from build123d import *

# Parameters (mm, degrees)
BOSS_EXTRUDE1_DEPTH     = 8
CUT_EXTRUDE1_START      = 8
CUT_EXTRUDE1_DEPTH      = 3
SKETCH1_12_R            = 1.7
CUT_EXTRUDE2_DEPTH      = 4
CUT_EXTRUDE3_DEPTH      = 230.948791245
CUT_EXTRUDE3_DEPTH_BACK = 230.948791245
SKETCH1_13_R            = 1.7


with BuildPart() as part:
    # Sketch1 → Boss-Extrude1 (new body)
    with BuildSketch(Plane(origin=(0, 0, 0), x_dir=(1, 0, 0), z_dir=(0, 1, 0))):
        with BuildLine():
            Line((97.462370633, 93.778736514), (-8.603646545, 168.04696129))
            ThreePointArc((-8.603646545, 168.04696129), (-12.287280664, 188.937888499), (8.603646545, 192.621522618))
            Line((8.603646545, 192.621522618), (114.669663723, 118.353297842))
            ThreePointArc((114.669663723, 118.353297842), (118.353297842, 97.462370633), (97.462370633, 93.778736514))
        make_face()
    extrude(amount=BOSS_EXTRUDE1_DEPTH)

    # Sketch1<11> → Cut-Extrude1 (cut)
    with BuildSketch(Plane(origin=(0, 0, 0), x_dir=(1, 0, 0), z_dir=(0, 1, 0)).offset(CUT_EXTRUDE1_START)):
        with BuildLine():
            Line((-15.839191899, 15.839191899), (90.226825279, 121.905209077))
            ThreePointArc((90.226825279, 121.905209077), (121.905209077, 121.905209077), (121.905209077, 90.226825279))
            Line((121.905209077, 90.226825279), (15.839191899, -15.839191899))
            ThreePointArc((15.839191899, -15.839191899), (-15.839191899, -15.839191899), (-15.839191899, 15.839191899))
        make_face()
    extrude(amount=-CUT_EXTRUDE1_DEPTH, mode=Mode.SUBTRACT)

    # Sketch1<12> → Cut-Extrude2 (cut)
    with BuildSketch(Plane(origin=(0, 0, 0), x_dir=(1, 0, 0), z_dir=(0, 1, 0))):
        with BuildLine():
            ThreePointArc((8.603646545, 192.621522618), (-9.076410828, 192.276551885), (-14.142135624, 175.334241954))
            Line((-14.142135624, 175.334241954), (33.292441968, 175.334241954))
            Line((33.292441968, 175.334241954), (8.603646545, 192.621522618))
        make_face()
        with Locations(Location((-9, 180.334241954, 0), (0, 0, 270))):
            Circle(SKETCH1_12_R, mode=Mode.SUBTRACT)
        with Locations(Location((0, 189.334241954, 0), (0, 0, 270))):
            Circle(SKETCH1_12_R, mode=Mode.SUBTRACT)
        with Locations(Location((9, 180.334241954, 0), (0, 0, 270))):
            Circle(SKETCH1_12_R, mode=Mode.SUBTRACT)
    extrude(amount=CUT_EXTRUDE2_DEPTH, mode=Mode.SUBTRACT)

    # Sketch1<13> → Cut-Extrude3 (cut, two sides: drawn at the far end of the back side and taken through both)
    with BuildSketch(Plane(origin=(0, 0, 0), x_dir=(1, 0, 0), z_dir=(0, 1, 0)).offset(-CUT_EXTRUDE3_DEPTH_BACK)):
        with Locations(Location((0, 189.334241954, 0), (0, 0, 270))):
            Circle(SKETCH1_13_R)
        with Locations(Location((-9, 180.334241954, 0), (0, 0, 270))):
            Circle(SKETCH1_13_R)
        with Locations(Location((9, 180.334241954, 0), (0, 0, 270))):
            Circle(SKETCH1_13_R)
        with Locations(Location((99.718863875, 119.666151183, 0), (0, 0, 270))):
            Circle(SKETCH1_13_R)
        with Locations(Location((91.11521733, 107.378870518, 0), (0, 0, 270))):
            Circle(SKETCH1_13_R)
        with Locations(Location((106.066017178, 106.066017178, 0), (0, 0, 270))):
            Circle(SKETCH1_13_R)
    extrude(amount=CUT_EXTRUDE3_DEPTH + CUT_EXTRUDE3_DEPTH_BACK, mode=Mode.SUBTRACT)


solid = part.part
Geometry: final body of the model. Coordinates: model frame, mm. A direction names the side the tool comes from. Give positions to 0.01 mm unless a question says otherwise; leave off trailing zeros. Loops run counter-clockwise (first coordinate to the right, second up) from the corner with the lowest first, then second, coordinate; pieces in that order, holes last. Notation, with made-up numbers: (-11.75, 33) - (13.25, 33) arc R18 ccw to (13.25, 47) - close; hole circle Ø3 at (-35, 3.5). An arc over 180 degrees is marked (long way). Answer as CSV lines item,"result". Start each with the question number.
1. Pin query (flat end, axial travel): P1, Ø2, axis at x = 91.12, z = -107.38, coming from the -Y side; P2, Ø2, axis at y = 6, z = -161.5, coming from the +X side; P3, Ø16, axis at x = -2, z = -186, coming from the -Y side; P4, Ø4, axis at x = 99.72, z = -119.67, coming from the +Y side. Return the tip coordinate at first contact, or that it passes through.
2. Section D-D, the plane x = 88. Return loops of the section in (y, z), plus the area to 3 significant figures.
3. Section C-C, the plane y = 2.75. Return loops of the section in (x, z), plus the area to 3 significant figures.
4. Section B-B, the plane z = -180.5. Return loops of the section in (x, y).
5. Section A-A, the plane x = 0. Return loops of the section in (y, z).
6. Ray query, L1, parallel to X at y = 4.5, z = -179; L2, parallel to Y at x = 6, z = -190; L3, parallel to Z at x = 0, y = 6.8. Return the intervals inside material, ascending.
7. Reachability of faces 1 (the face through (100.868, 2.465, -120.919)), 2 (the face through (104, 5, -110)), 3 (the face through (9, 2, -175.334)) from +Z, -Z, +X, -X, +Y, -Y: full face, straight path, thin tool, end or side. Return the list, or none.
Answers:
1,P1,"passes through"
1,P2,"stops at x = 54.48"
1,P3,"stops at y = 4"
1,P4,"stops at y = 5"
2,outline,"(0, -137.03) - (8, -137.03) - (8, -119.68) - (5, -119.68) - (5, -100.4) - (0, -100.4) - close"
2,area,"235 mm2"
3,outline,"(-14.14, -175.33) - (33.29, -175.33) - (114.67, -118.35) arc R15 ccw to (97.46, -93.78) - (-8.6, -168.05) arc R15 ccw to start; hole circle Ø3.4 at (91.12, -107.38); hole circle Ø3.4 at (99.72, -119.67); hole circle Ø3.4 at (106.07, -106.07)"
3,area,"3,940 mm2"
4,outline,"(-15, 4) - (-10.69, 4) - (-10.69, 8) - (-15, 8) - close; (-7.31, 4) - (7.31, 4) - (7.31, 8) - (-7.31, 8) - close; (10.69, 4) - (25.91, 4) - (25.91, 8) - (10.69, 8) - close"
5,outline,"(0, -175.33) - (4, -175.33) - (4, -187.63) - (8, -187.63) - (8, -162.02) - (0, -162.02) - close; (4, -195.33) - (8, -195.33) - (8, -191.03) - (4, -191.03) - close"
6,L1,"x = -14.94 to -10.05, -7.95 to 7.95, 10.05 to 28.06"
6,L2,"y = 4 to 8"
6,L3,"z = -195.33 to -191.03, -187.63 to -162.02"
7,face 1,"+Y, -Y"
7,face 2,"+Z, +X, +Y"
7,face 3,"-Z, +X, -X, -Y"
